from build123d import *

# Parameters (mm, degrees)
F1_DEPTH      = 76.2
F2_W          = 139.7
F2_H          = 36.3417792003
F3_DEPTH      = 25.4
F7_DEPTH      = 27.275979542
F7_DEPTH_BACK = 66.7271380179
F9_DEPTH      = 66.7271380179


with BuildPart() as f1:
    # F0 (on Right) → F1 (new body, symmetric)
    with BuildSketch(Plane.YZ):
        with BuildLine():
            ThreePointArc((-0.2200527473, 12.7), (-9.7450527473, 3.175), (-19.2700527473, 12.7))
            Line((-19.2700527473, 12.7), (-22.4450527473, 12.7))
            ThreePointArc((-22.4450527473, 12.7), (-18.7253088684, 3.7197438789), (-9.7450527473, 0))
            Line((-9.7450527473, 0), (-2.4182328489, 0))
            Line((-2.4182328489, 0), (-2.4182328489, 2.3265863779))
            ThreePointArc((-2.4182328489, 2.3265863779), (-1.4157111092, 3.1129218281), (-0.4970236472, 3.9957505917))
            ThreePointArc((-0.4970236472, 3.9957505917), (0.3027257677, 2.6962087261), (1.3655856019, 1.6013401678))
            Line((1.3655856019, 1.6013401678), (1.3655856019, 0))
            Line((1.3655856019, 0), (9.7478376701, 0))
            Line((9.7478376701, 0), (9.7478376701, 1.2116913596))
            ThreePointArc((9.7478376701, 1.2116913596), (10.4868542157, 1.7913884), (11.1414158123, 2.4649930537))
            ThreePointArc((11.1414158123, 2.4649930537), (11.784015325, 1.75263856), (12.5265968964, 1.145221349))
            Line((12.5265968964, 1.145221349), (12.5265968964, 0))
            Line((12.5265968964, 0), (16.1642856123, 0))
            Line((16.1642856123, 0), (71.5560648125, 0))
            Line((71.5560648125, 0), (71.5560648125, 6.35))
            ThreePointArc((71.5560648125, 6.35), (71.3396938095, 7.9935009364), (70.7053261266, 9.525))
            Line((70.7053261266, 9.525), (37.2091680094, 67.5420477173))
            ThreePointArc((37.2091680094, 67.5420477173), (30.8810653748, 70.662722587), (25.5762776984, 66.0105486537))
            Line((25.5762776984, 66.0105486537), (9.4962047547, 5.9988994382))
            ThreePointArc((9.4962047547, 5.9988994382), (4.8299267947, 3.3048226018), (2.1358499583, 7.9711005618))
            Line((2.1358499583, 7.9711005618), (3.4029547439, 12.7))
            Line((3.4029547439, 12.7), (-0.2200527473, 12.7))
        make_face()
        with BuildLine():
            ThreePointArc((67.9556954695, 7.9375), (67.9556954695, 4.7625), (65.2060648125, 3.175))
            Line((65.2060648125, 3.175), (16.1642856123, 3.175))
            ThreePointArc((16.1642856123, 3.175), (13.6453887568, 4.4171824629), (13.0974711138, 7.1717504682))
            Line((13.0974711138, 7.1717504682), (28.6430921969, 65.1887981855))
            ThreePointArc((28.6430921969, 65.1887981855), (31.2954860351, 67.5148851522), (34.4595373524, 65.9545477173))
            Line((34.4595373524, 65.9545477173), (67.9556954695, 7.9375))
        make_face(mode=Mode.SUBTRACT)
    extrude(amount=F1_DEPTH, both=True)

    # F2 (on face) → F3 (cut)
    with BuildSketch(Plane.XY.offset(3.175)):
        with Locations((0, 40.6851752124)):
            Rectangle(F2_W, F2_H)
    extrude(amount=-F3_DEPTH, mode=Mode.SUBTRACT)

    # F6 (on plane+point) → F7 (cut, two sides)
    with BuildSketch(Plane.XZ.offset(-4.8299267947)) as f7_sk:
        Polygon((76.2, 73.3377320159), (6.0372679841, 73.3377320159), (76.2, 3.175), align=None)
        Polygon((-76.2, 3.175), (-6.0372679841, 73.3377320159), (-76.2, 73.3377320159), align=None)
    extrude(amount=F7_DEPTH, mode=Mode.SUBTRACT)
    extrude(f7_sk.sketch, amount=-F7_DEPTH_BACK, mode=Mode.SUBTRACT)

    # F8 (on plane+point) → F9 (cut, through all)
    with BuildSketch(Plane.XZ.offset(-4.8299267947)):
        with BuildLine():
            Line((-5.499261314, 64.5894877579), (-40.9569323532, 3.175))
            Line((-40.9569323532, 3.175), (40.9569323532, 3.175))
            Line((40.9569323532, 3.175), (5.499261314, 64.5894877579))
            ThreePointArc((5.499261314, 64.5894877579), (0, 67.7644877579), (-5.499261314, 64.5894877579))
        make_face()
    extrude(amount=-F9_DEPTH, mode=Mode.SUBTRACT)


solid = f1.part
Design review of the part built by this model. Coordinates are the model's own, in mm. A direction names the side the tool comes from. Give positions to 0.01 mm unless a question says otherwise; leave off trailing zeros. Loops run counter-clockwise (first coordinate to the right, second up) from the corner with the lowest first, then second, coordinate; pieces in that order, holes last. Notation, with made-up numbers: (-38.5, -13.5) - (-15.5, -13.5) arc R26 cw to (-15.5, 12.5) - close; hole circle Ø10 at (82.25, 12). An arc over 180 degrees is marked (long way). Write item = value, one per line.
1) Clearance check with flat-ended pins moving along their axes: pin 1 Ø0.9 at (x, z) = (15.5, 0.5) entering from -Y; pin 2 Ø2.5 at (x, z) = (4.5, 1) entering from -Y; pin 3 Ø1.1 at (x, y) = (-30, 1.5) entering from +Z; pin 4 Ø3 at (x, y) = (-38, 2) entering from -Z. State where each tip first meets the part, or that it passes through.
Result sheet:
pin_1 = -14.56
pin_2 = -16.96
pin_3 = 12.7
pin_4 = 0
2) Take a section at A-A on z = 46. State the section outline as (x, y) points (3 decimals), and give its area (3 significant figures).
Result sheet:
outline = (-33.375, 20.214) - (-16.232, 20.214) - (-16.232, 23.501) - (-33.375, 23.501) - close; (-33.375, 45.98) - (-16.232, 45.98) - (-16.232, 49.646) - (-33.375, 49.646) - close; (16.232, 20.214) - (33.375, 20.214) - (33.375, 23.501) - (16.232, 23.501) - close; (16.232, 45.98) - (33.375, 45.98) - (33.375, 49.646) - (16.232, 49.646) - close
area = 238 mm2
3) Take a section at B-B on x = -19. Count the separate pieces of the cut face and the enclosed holes in it, and give its area (3 significant figures).
Result sheet:
separate_pieces = 4
enclosed_holes = 0
area = 363 mm2
4) Tool access review of faces 1 (the face through (-1, 22.514, 2)), 2 (the face through (-32.8, 53.6, 32.8)), 3 (the face through (69.85, 40, 2)): name each direction out of +Z, -Z, +X, -X, +Y, -Y from which nothing blocks a thin tool from reaching the whole face with its end or side.
Result sheet:
face_1 = -Z
face_2 = +X, -X
face_3 = +Z, -Z
5) Take a section at C-C on z = 28.5. State the section outline as (x, y) points (3 decimals).
Result sheet:
outline = (-50.875, 15.525) - (-26.336, 15.525) - (-26.336, 18.812) - (-50.875, 18.812) - close; (-50.875, 56.084) - (-26.336, 56.084) - (-26.336, 59.75) - (-50.875, 59.75) - close; (26.336, 15.525) - (50.875, 15.525) - (50.875, 18.812) - (26.336, 18.812) - close; (26.336, 56.084) - (50.875, 56.084) - (50.875, 59.75) - (26.336, 59.75) - close
6) Draft analysis for pull direction Y (two halves, no side actions). For faces 4 (the face through (0.187, 30.985, 70.676)), 5 (the face through (-5, 21, 3.175)), 6 (the face through (1.067, -18.824, 3.819)), 7 (the face through (-72.165, -18.888, 7.21)), state which applies: +Y half, -Y half, draft (parallel to the pull), parting line (faces both ways), or undercut.
Result sheet:
face_4 = parting line
face_5 = undercut
face_6 = -Y half
face_7 = draft
7) To check wall thickness, follow line 1 (Y direction, x = -45, z = 7); line 2 (Y direction, x = 30, z = 29); line 3 (Z direction, x = 69, y = 60.5) (3 decimals). State the ranges of each line that lie inside material, in increasing order.
Result sheet:
line_1 = -21.09 to -17.38, -2.11 to 2.01, 9.76 to 13.06, 68.31 to 71.52
line_2 = 15.66 to 18.95, 55.8 to 59.46
line_3 = 0 to 3.175
